Print and shaded views of the part. All mm, measured from the part's lowest x, y and z. A direction names the side the tool comes from. Coordinates: 2 decimals unless noted, no trailing zeros. Order: outer loops, then holes, each group sorted by start corner. A loop starts at its lowest first (then second) coordinate and runs counter-clockwise, first axis right, second up. Notation, with made-up numbers: (31.5, 73) -> (39.5, 73) arc R6 cw to (39.5, 84) -> close; hole circle Ø1 at (-23, 22). An arc over 180 degrees is marked (long way). Return JSON: item names as keys, results as strings. Group by question number.
1) Cut at A-A (z = 89.5). Write the cut outline in (x, y).
2) Which spindle directions (+Z, -Z, +X, -X, +Y, -Y) get a long thin tool onto all of the face, cutting with end or side? Do the marked faces 4 and 5. Say none if no direction does.
3) Cut at B-B (y = 130). Write the cut outline in (x, z).
4) Cut at C-C (x = 217). Write the cut outline in (y, z), and give its area (3 significant figures).
5) Probe line 1 (X direction, y = 234, z = 66); line 2 (Y direction, x = 79, z = 215.5). List the from-to ranges inside material, lowest first.
6) Pull direction Y, two halves, no side cores. Call the marked faces 1, 2 and 3: +Y half, -Y half, draft (parallel to the pull), parting line (faces both ways), or undercut.
7) Flat gauge pins, fed straight in: pin 1 (8 mm diameter, centred on x = 10, y = 234, fed in from -Z); pin 2 (6 mm diameter, centred on x = 177.5, y = 175.5, fed in from -Z). Where does each tip first touch, or does it go through?
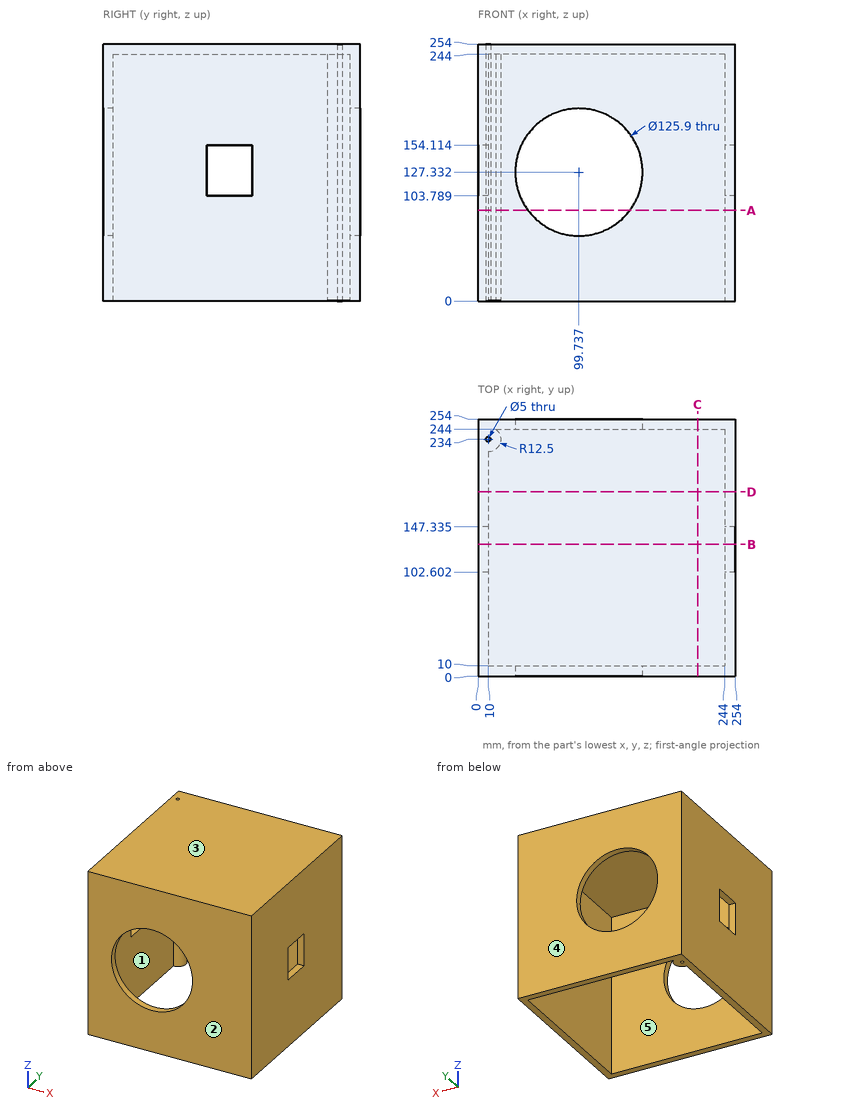
Answers below:
{
 "1": {"outline": "(0, 0) -> (49.42, 0) -> (49.42, 10) -> (10, 10) -> (10, 221.5) arc R12.5 ccw to (17.5, 244) -> (49.42, 244) -> (49.42, 254) -> (0, 254) -> close; (150.05, 0) -> (254, 0) -> (254, 254) -> (150.05, 254) -> (150.05, 244) -> (244, 244) -> (244, 10) -> (150.05, 10) -> close; hole circle Ø5 at (10, 234)"},
 "2": {"face 4": "+Z, -Z, +X, -X, +Y", "face 5": "-Z"},
 "3": {"outline": "(0, 0) -> (10, 0) -> (10, 103.79) -> (0, 103.79) -> close; (0, 154.11) -> (10, 154.11) -> (10, 244) -> (244, 244) -> (244, 154.11) -> (254, 154.11) -> (254, 254) -> (0, 254) -> close; (244, 0) -> (254, 0) -> (254, 103.79) -> (244, 103.79) -> close"},
 "4": {"outline": "(0, 0) -> (10, 0) -> (10, 244) -> (244, 244) -> (244, 0) -> (254, 0) -> (254, 254) -> (0, 254) -> close", "area": "7,420 mm^2"},
 "5": {"line 1": "x = 0 to 7.5, 12.5 to 22.5, 244 to 254", "line 2": "y = 0 to 10, 244 to 254"},
 "6": {"face 1": "undercut", "face 2": "-Y half", "face 3": "draft"},
 "7": {"pin 1": "stops at z = 0", "pin 2": "stops at z = 244"}
}
